The figure shows three views and two pictorial views of one solid part (mm, origin at its lowest corner). Answer the questions. A direction names the side the tool comes from. Coordinates: 2 decimals unless noted, no trailing zeros. Order: outer loops, then holes, each group sorted by start corner. A loop starts at its lowest first (then second) coordinate and runs counter-clockwise, first axis right, second up. Notation, with made-up numbers: (10, -13) -> (42, -13) arc R29 cw to (42, 13) -> close; hole circle Ø1 at (73.25, 0). An arc over 180 degrees is marked (long way). Write item = value, one per line.
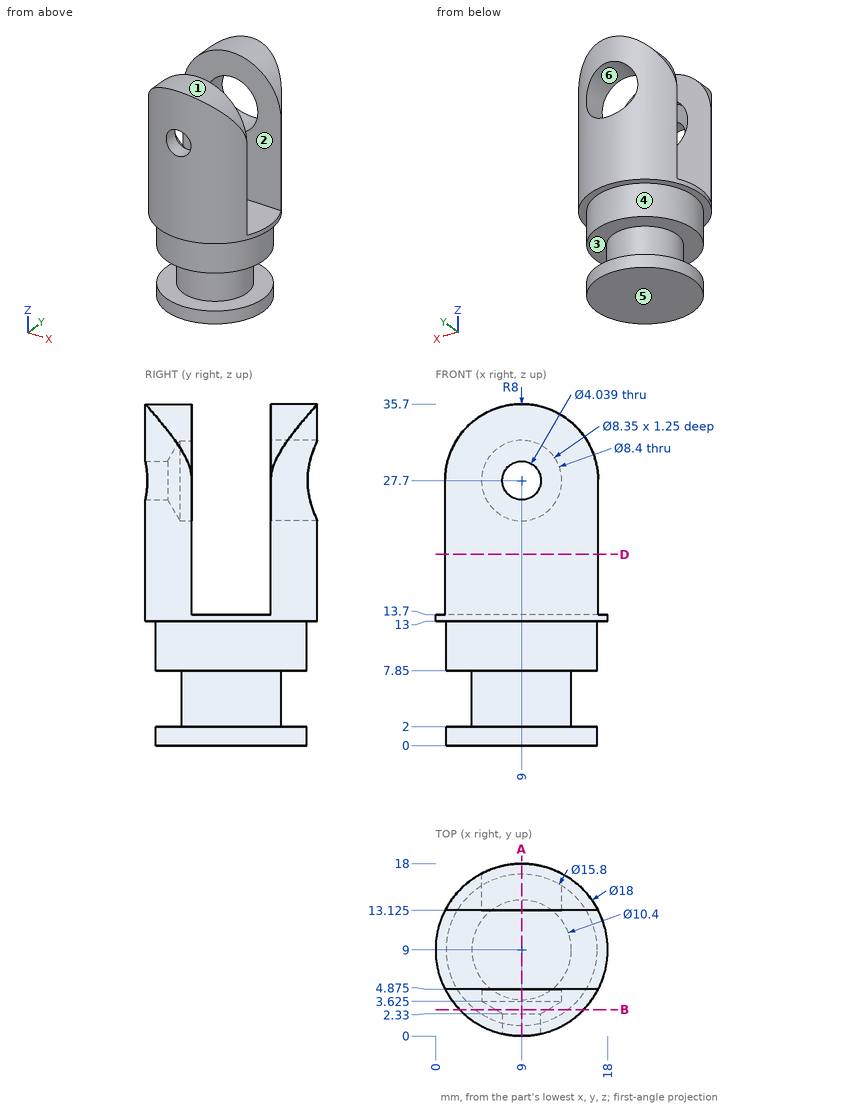
Q1. Find the intervals of material crossed by line 1 along Z through (x, y) = (9, 15.75); line 2 along Z through (x, y) = (9, 4.05) (1 decimal); line 3 along Z through (x, y) = (9, 1.05), in increasing order.
The answers:
line_1 = 0 to 2, 7.85 to 23.5, 31.9 to 35.7
line_2 = 0 to 23.5, 31.9 to 35.7
line_3 = 13 to 25.68, 29.72 to 35.7
Q2. Section A-A, the plane x = 9 is taken. Give the number of separate pieces and of enclosed holes in the cut face, plus the area to 3 significant figures.
The answers:
separate_pieces = 3
enclosed_holes = 0
area = 332 mm2
Q3. Section B-B, the plane y = 2.75 is taken. Give the vertices of the cut face in (x, z).
The answers:
outline = (2.52, 13) -> (4.17, 13) -> (4.17, 7.85) -> (13.83, 7.85) -> (13.83, 13) -> (15.48, 13) -> (15.48, 32.4) arc R8 ccw to (2.52, 32.4) -> close; (4.17, 0) -> (13.83, 0) -> (13.83, 2) -> (4.17, 2) -> close; hole circle Ø5.44 at (9, 27.7)
Q4. The mould has two halves that part along X. Classify the marked faces 4, 5 and 6: released by +X, released by -X, zero draft, split by the parting line, or undercut.
The answers:
face_4 = split by the parting line
face_5 = zero draft
face_6 = undercut
Q5. Each of these flat-tipped pins is pushed along its axis until it touches: pin 1 Ø4 at (x, z) = (16, 8) entering from -Y (1 decimal); pin 2 Ø2 at (x, y) = (6, 10.5) entering from +Z; pin 3 Ø2 at (y, z) = (12, 27) entering from +X; pin 4 Ø5 at (x, y) = (13, 14) entering from -Z. Where does it stop, or does it pass through?
The answers:
pin_1 = 2.9
pin_2 = 13.7
pin_3 = through
pin_4 = 0
Q6. Section D-D, the plane z = 20 is taken. Give the vertices of the cut face in (x, y) (1 decimal), plus the area to 3 significant figures.
The answers:
outline = (1, 4.9) arc R9 ccw to (17, 4.9) -> close; (1, 13.1) -> (17, 13.1) arc R9 ccw to start
area = 111 mm2
Q7. A tool of negligible diameter and unlimited length cuts with its end or side. For the marked faces 1, 2 and 3, from which of +Z, -Z, +X, -X, +Y, -Y can it reach the whole face along a straight path? Write none if from no direction.
The answers:
face_1 = +Z, +Y, -Y
face_2 = +Z, +X, -X
face_3 = none
